Verification items for the finished model (mm, model axes). Coordinates: 2 decimals unless noted, no trailing zeros. Order: outer loops, then holes, each group sorted by start corner. A loop starts at its lowest first (then second) coordinate and runs counter-clockwise, first axis right, second up. Notation, with made-up numbers: M -15.75,-33.5 L 42.25,-33.5 A31 cw 42.25,-3.5 Z; hole C 45,28 d7. An arc over 180 degrees is marked long. Write item = value, one per line.
```python
from build123d import *

# Parameters (mm, degrees)
SKETCH2_W           = 100
SKETCH2_H           = 200
BOSS_EXTRUDE1_DEPTH = 1.5
SKETCH4_R           = 2.667
CUT_EXTRUDE1_DEPTH  = 2
SKETCH5_R           = 2.667
SKETCH5_R_2         = 1.5
BOSS_EXTRUDE2_DEPTH = 0.254
SKETCH6_W           = 7.5
SKETCH6_H           = 150
CUT_EXTRUDE2_DEPTH  = 1.5
SKETCH7_W           = 7.5
SKETCH7_H           = 1.5
CUT_EXTRUDE3_DEPTH  = 1.5


with BuildPart() as part:
    # Sketch2 → Boss-Extrude1 (new body)
    with BuildSketch(Plane.XY):
        with Locations((50, 100)):
            Rectangle(SKETCH2_W, SKETCH2_H)
    extrude(amount=BOSS_EXTRUDE1_DEPTH)

    # Sketch4 → Cut-Extrude1 (cut)
    with BuildSketch(Plane.XY.offset(1.5)):
        with Locations((4, 195)):
            Circle(SKETCH4_R)
        with Locations((96, 195)):
            Circle(SKETCH4_R)
        with Locations((96, 5)):
            Circle(SKETCH4_R)
        with Locations((4, 5)):
            Circle(SKETCH4_R)
    extrude(amount=-CUT_EXTRUDE1_DEPTH, mode=Mode.SUBTRACT)

    # Sketch5 → Boss-Extrude2 (add)
    # profile 1 of 4: a face of its own
    with BuildSketch(Plane.XY.offset(1.5)):
        with Locations((3.959685834, 5.068811707)):
            Circle(SKETCH5_R)
        with Locations(Location((3.959685834, 5.068811707, 0), (0, 0, 180))):
            Circle(SKETCH5_R_2, mode=Mode.SUBTRACT)
    # profile 2 of 4: a face of its own
    with BuildSketch(Plane.XY.offset(1.5)):
        with Locations((3.959685834, 194.931188293)):
            Circle(SKETCH5_R)
        with Locations((3.959685834, 194.931188293)):
            Circle(SKETCH5_R_2, mode=Mode.SUBTRACT)
    # profile 3 of 4: a face of its own
    with BuildSketch(Plane.XY.offset(1.5)):
        with Locations((96.040314166, 5.068811707)):
            Circle(SKETCH5_R)
        with Locations((96.040314166, 5.068811707)):
            Circle(SKETCH5_R_2, mode=Mode.SUBTRACT)
    # profile 4 of 4: a face of its own
    with BuildSketch(Plane.XY.offset(1.5)):
        with Locations((96.040314166, 194.931188293)):
            Circle(SKETCH5_R)
        with Locations(Location((96.040314166, 194.931188293, 0), (0, 0, 180))):
            Circle(SKETCH5_R_2, mode=Mode.SUBTRACT)
    extrude(amount=-BOSS_EXTRUDE2_DEPTH)

    # Sketch6 → Cut-Extrude2 (cut)
    with BuildSketch(Plane.XY):
        with Locations((3.75, 100)):
            Rectangle(SKETCH6_W, SKETCH6_H)
        with Locations((96.25, 100)):
            Rectangle(SKETCH6_W, SKETCH6_H)
    extrude(amount=CUT_EXTRUDE2_DEPTH, mode=Mode.SUBTRACT)

    # Sketch7 → Cut-Extrude3 (cut)
    with BuildSketch(Plane.XZ.offset(-175)):
        with Locations((3.75, 0.75)):
            Rectangle(SKETCH7_W, SKETCH7_H)
        with Locations((96.25, 0.75)):
            Rectangle(SKETCH7_W, SKETCH7_H)
    extrude(amount=-CUT_EXTRUDE3_DEPTH, mode=Mode.SUBTRACT)


solid = part.part
```
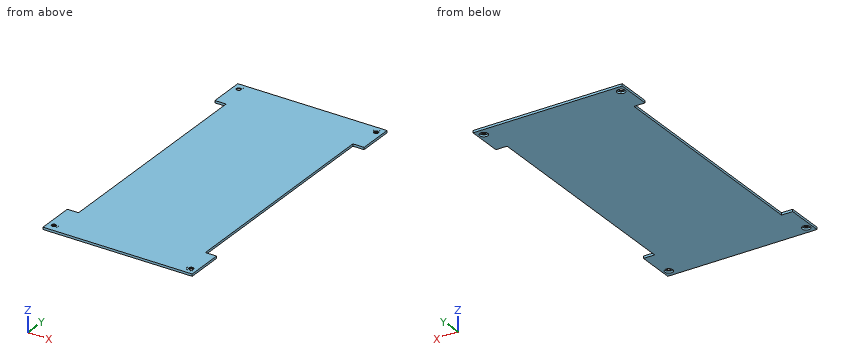
Item 1: Gauge pin test, flat end, axial feed: pin 1 (2.5 mm diameter, centred on x = 97, y = 194.5, fed in from -Z). Record the tip position at first contact, or that the pin passes through.
Report:
pin_1 = 1.25
Item 2: Sectioned sample at A-A, the plane z = 0.85. Enter the section's corners in (x, y), then the cut area to 3 significant figures.
Report:
outline = M 0,0 L 100,0 L 100,25 L 92.5,25 L 92.5,176.5 L 100,176.5 L 100,200 L 0,200 L 0,176.5 L 7.5,176.5 L 7.5,25 L 0,25 Z; hole C 4,5 d5.33; hole C 4,195 d5.33; hole C 96,5 d5.33; hole C 96,195 d5.33
area = 17,600 mm^2
Item 3: Sectioned sample at B-B, the plane y = 127. Enter the section's corners in (x, z), then the cut area to 4 significant figures.
Report:
outline = M 7.5,0 L 92.5,0 L 92.5,1.5 L 7.5,1.5 Z
area = 127.5 mm^2
Item 4: Scan lines: L1, parallel to Y at x = 4, z = 0.3; L2, parallel to X at y = 195, z = 0.35; L3, parallel to Y at x = 93, z = 0.95. Record each from-to range of solid material in increasing order. Write a range as from..to.
Report:
L1 = 0..2.33, 7.67..25, 176.5..192.33, 197.67..200
L2 = 0..1.33, 6.67..93.33, 98.67..100
L3 = 0..25, 176.5..200
